Solid Edge part; units mm, degrees
sketch "Sketch1" plane through (0, 0, 0) normal (0, 0, 1) x (1, 0, 0)
  line L0 (-7.5, 0) -> (-7.5, 9.5)
  line L1 (-7.5, 9.5) -> (-6.6828, 12.55)
  line L2 (-6.6828, 12.55) -> (-0.5, 12.55)
  line L3 (-0.5, 12.55) -> (-0.5, 8.3)
  line L4 (-0.5, 8.3) -> (0, 8.3)
  line L5 (0, 8.3) -> (0, 6)
  line L6 (0, 6) -> (48.9265, 6)
  line L7 (48.9265, 6) -> (50, 4.9265)
  line L8 (50, 4.9265) -> (50, 0)
  line L9 (50, 0) -> (-7.5, 0)
revolve "RevolvedProtrusion1" add sketch "Sketch1" angle 360 about axis through (50, 0, 0) along (-1, 0, 0)
cosmetic_thread "Thread1"
sketch "Sketch2" plane through (-7.5, 0, 0) normal (-1, 0, 0) x (0, -1, 0)
  circle A0 centre (0, 0) radius 14.55
  line L0 (9.5, 5.4848) -> (0, 10.9697)
  line L1 (0, 10.9697) -> (-9.5, 5.4848)
  line L2 (-9.5, 5.4848) -> (-9.5, -5.4848)
  line L3 (-9.5, -5.4848) -> (0, -10.9697)
  line L4 (0, -10.9697) -> (9.5, -5.4848)
  line L5 (9.5, -5.4848) -> (9.5, 5.4848)
extrude "ExtrudedCutout_1" cut sketch "Sketch2" against normal blind 7.5
properties part number "07171-12X50"
Read the model definition and answer for the solid it produces. Units are mm, in the model's axes. A direction names the side the tool comes from. Coordinates: 2 decimals unless noted, no trailing zeros. Loops run counter-clockwise (first coordinate to the right, second up) from the corner with the lowest first, then second, coordinate; pieces in that order, holes last.
Q1. Which of the six approach directions +Z, -Z, +X, -X, +Y, -Y give full straight-line access (tool end or side, diameter ignored) to faces 1 (the face through (-7.5, 0, 0)), 2 (the face through (0, -2, -6))?
Q2. Each of these flat-tipped pins is pushed along its axis until it touches: pin 1 Ø3 at (x, y) = (2.5, 4) entering from +Z; pin 2 Ø10 at (x, z) = (26, 6.5) entering from -Y; pin 3 Ø3 at (x, y) = (34.5, 2) entering from +Z. Where does it stop, or does it pass through?
Q3. The part is cut by section A-A on x = 38. Write down the section's boundary in (y, z), and give its area (3 significant figures).
Q4. Consider probe 1 along X at (y, z) = (-6.75, -2.5); probe 2 along Z at (x, y) = (42, 0.25); probe 3 along X at (y, z) = (1.25, -8.25). Determine where each line is inside the solid, lowest interval first.
Results below:
1. face 1: +Z, -Z, -X, +Y, -Y
1. face 2: +X
2. pin 1: stops at z = 5.45
2. pin 2: stops at y = -5.81
2. pin 3: stops at z = 5.98
3. outline: circle Ø12 at (0, 0)
3. area: 113 mm2
4. probe 1: x = -7.5 to 0
4. probe 2: z = -5.99 to 5.99
4. probe 3: x = -7.5 to -0.5
